```python
from build123d import *

# Parameters (mm, degrees)
BOSS_EXTRUDE1_DEPTH = 48
SKETCH4_W           = 48
SKETCH4_H           = 48
SKETCH4_W_2         = 42
SKETCH4_H_2         = 42
BOSS_EXTRUDE2_DEPTH = 25
SKETCH5_W           = 42
SKETCH5_H           = 42
BOSS_EXTRUDE3_DEPTH = 3
SKETCH7_R           = 3.4
CUT_EXTRUDE1_DEPTH  = 99.707699801
SKETCH8_W           = 30
SKETCH8_H           = 25
CUT_EXTRUDE3_DEPTH  = 10
BOSS_EXTRUDE4_DEPTH = 3


with BuildPart() as part:
    # Sketch3 → Boss-Extrude1 (new body)
    with BuildSketch(Plane(origin=(0, 0, 0), x_dir=(0, 0, -1), z_dir=(1, 0, 0))):
        Polygon((0, 0), (0, 5), (24, 5), (24, 7), (-2, 7), (-2, 2), (-83.9, 2), (-83.9, 0), align=None)
    extrude(amount=BOSS_EXTRUDE1_DEPTH)

    # Sketch4 → Boss-Extrude2 (add)
    with BuildSketch(Plane(origin=(0, 2, 0), x_dir=(1, 0, 0), z_dir=(0, 1, 0))):
        with Locations((24, -59.9)):
            Rectangle(SKETCH4_W, SKETCH4_H)
        with Locations((24, -59.9)):
            Rectangle(SKETCH4_W_2, SKETCH4_H_2, mode=Mode.SUBTRACT)
    extrude(amount=BOSS_EXTRUDE2_DEPTH)

    # Sketch5 → Boss-Extrude3 (add)
    with BuildSketch(Plane(origin=(0, 2, 0), x_dir=(1, 0, 0), z_dir=(0, 1, 0))):
        with Locations((24, -59.9)):
            Rectangle(SKETCH5_W, SKETCH5_H)
    extrude(amount=BOSS_EXTRUDE3_DEPTH)

    # Sketch7 → Cut-Extrude1 (cut, through all)
    with BuildSketch(Plane(origin=(0, 7, 0), x_dir=(1, 0, 0), z_dir=(0, 1, 0))):
        with Locations(Location((11, 18, 0), (0, 0, 270))):
            Circle(SKETCH7_R)
        with Locations(Location((37, 18, 0), (0, 0, 270))):
            Circle(SKETCH7_R)
    extrude(amount=-CUT_EXTRUDE1_DEPTH, mode=Mode.SUBTRACT)

    # Sketch8 → Cut-Extrude3 (cut)
    with BuildSketch(Plane(origin=(0, 0, 35.9), x_dir=(-1, 0, 0), z_dir=(0, 0, -1))):
        with Locations((-24, 14.5)):
            Rectangle(SKETCH8_W, SKETCH8_H)
    extrude(amount=-CUT_EXTRUDE3_DEPTH, mode=Mode.SUBTRACT)

    # Sketch9 → Boss-Extrude4 (add)
    with BuildSketch(Plane(origin=(0, 2, 0), x_dir=(1, 0, 0), z_dir=(0, 1, 0))):
        Polygon((0, -2), (0, -35.9), (9, -35.9), (9, -45.9), (39, -45.9), (39, -35.9), (48, -35.9), (48, -2), align=None)
    extrude(amount=BOSS_EXTRUDE4_DEPTH)


solid = part.part
```
Model file for the job. Use its own axes, mm. A direction names the side the tool comes from. Give positions to 0.01 mm unless a question says otherwise; leave off trailing zeros. Write each loop counter-clockwise with the first axis right and the second up, starting at its lowest first coordinate (ties: lowest second). Pieces come first, ordered by that corner, then holes. Notation, with made-up numbers: (59.5, 76) - (117.5, 76) arc R31 cw to (117.5, 107) - close; hole circle Ø7 at (30, 32). An arc over 180 degrees is marked (long way). One line per question, with ' | ' between items. Start each with the question number.
(1) Slice it at A-A on x = 37. Write the cut outline in (y, z).
(2) Slice it at C-C on y = 25. Write the cut outline in (x, z).
(3) Slice it at B-B on z = 62.5. Write the cut outline in (x, y).
(4) Two-plate mould, pull along Z, no slides. Class faces 1 (the face through (24, 0, 43)), 2 (the face through (24, 13, 83.9)), 3 (the face through (3, 16, 60)), 4 (the face through (24, 2, 0)): +Z half, -Z half, draft (parallel to the pull), parting line (faces both ways), or undercut.
(5) 3-axis set-ups, long thin cutter, end or side, ignore diameter. For faces 5 (the face through (24, 6, 2)), 6 (the face through (42, 16, 38.9)), 7 (the face through (24, 7, -11)): which of +Z, -Z, +X, -X, +Y, -Y reach the whole face in a straight line?
(6) Wall check: line 1 along X through (y, z) = (5.8, -18); line 2 along Z through (x, y) = (4.5, 6); line 3 along X through (y, z) = (5.25, 39). Give the ranges that are in metal, low to high. Write a range as from..to.
(7) Pin check, flat tips, straight feed: P1, Ø8, axis at x = 6, z = 29.5, coming from the +Y side; P2, Ø1, axis at x = 27, y = 10, coming from the -Z side; P3, Ø7, axis at x = 42, y = 20, coming from the -Z side. Stop position of each tip, or through.
(8) Slice it at D-D on z = -18. Write the cut outline in (x, y), plus the area to 3 significant figures.
Results below:
1) outline: (0, 0) - (5, 0) - (5, -14.6) - (7, -14.6) - (7, 2) - (5, 2) - (5, 80.9) - (27, 80.9) - (27, 83.9) - (0, 83.9) - close; (5, -24) - (7, -24) - (7, -21.4) - (5, -21.4) - close
2) outline: (0, 35.9) - (9, 35.9) - (9, 38.9) - (3, 38.9) - (3, 80.9) - (45, 80.9) - (45, 38.9) - (39, 38.9) - (39, 35.9) - (48, 35.9) - (48, 83.9) - (0, 83.9) - close
3) outline: (0, 0) - (48, 0) - (48, 27) - (45, 27) - (45, 5) - (3, 5) - (3, 27) - (0, 27) - close
4) face 1: draft | face 2: +Z half | face 3: undercut | face 4: -Z half
5) face 5: +X, -X, +Y | face 6: +Y | face 7: -Z, +X, -X, +Y
6) line 1: 0..7.6, 14.4..33.6, 40.4..48 | line 2: -24..2, 35.9..38.9, 80.9..83.9 | line 3: 0..3, 45..48
7) P1: y = 5 | P2: z = 80.9 | P3: z = 35.9
8) outline: (0, 5) - (7.6, 5) - (7.6, 7) - (0, 7) - close; (14.4, 5) - (33.6, 5) - (33.6, 7) - (14.4, 7) - close; (40.4, 5) - (48, 5) - (48, 7) - (40.4, 7) - close | area: 68.8 mm^2
